The listing builds one solid part. Answer for the finished solid, in the listing's coordinates (mm). A direction names the side the tool comes from. Coordinates: 2 decimals unless noted, no trailing zeros. Write each loop counter-clockwise with the first axis right and the second up, starting at its lowest first coordinate (ties: lowest second). Pieces come first, ordered by that corner, then holes. Notation, with made-up numbers: M 70.5,35 L 111.5,35 A20 ccw 111.5,49 Z; hole C 16,-24 d11. An arc over 180 degrees is marked long. Put each result on its own line as item: value. Start each with the question number.
```python
from build123d import *

# Parameters (mm, degrees)
SKETCH1_W            = 25
SKETCH1_H            = 25
SKETCH1_W_2          = 9
SKETCH1_H_2          = 21
BOSS_EXTRUDE1_DEPTH  = 1.5
BOSS_EXTRUDE2_DEPTH  = 2
BOSS_EXTRUDE3_DEPTH  = 2
BOSS_EXTRUDE8_DEPTH  = 2
SKETCH12_W           = 2
SKETCH12_H           = 25
BOSS_EXTRUDE10_DEPTH = 5.93
SKETCH11_W           = 18
SKETCH11_H           = 25
SKETCH11_W_2         = 14
SKETCH11_H_2         = 21
BOSS_EXTRUDE11_DEPTH = 2
SKETCH13_W           = 9
SKETCH13_H           = 3.93
CUT_EXTRUDE2_DEPTH   = 24.5


with BuildPart() as part:
    # Sketch1 → Boss-Extrude1 (new body)
    with BuildSketch(Plane(origin=(0, 0, 0), x_dir=(1, 0, 0), z_dir=(0, 1, 0))):
        with Locations((0, -1)):
            Rectangle(SKETCH1_W, SKETCH1_H)
        with Locations((-6, -1)):
            Rectangle(SKETCH1_W_2, SKETCH1_H_2, mode=Mode.SUBTRACT)
        with Locations((6, -1)):
            Rectangle(SKETCH1_W_2, SKETCH1_H_2, mode=Mode.SUBTRACT)
    extrude(amount=BOSS_EXTRUDE1_DEPTH)

    # Sketch2 → Boss-Extrude2 (add)
    with BuildSketch(Plane(origin=(12.5, 0, 0), x_dir=(0, 0, -1), z_dir=(1, 0, 0))):
        Polygon((-9.5, 7.5), (-1, 7.5), (-1, 0), (1, 0), (1, 7.5), (7.5, 7.5), (7.5, 0), (11.5, 0), (11.5, 9.5), (-13.5, 9.5), (-13.5, 0), (-9.5, 0), align=None)
    extrude(amount=BOSS_EXTRUDE2_DEPTH)

    # Sketch3 → Boss-Extrude3 (add)
    with BuildSketch(Plane.ZY.offset(12.5)):
        Polygon((1, 0), (1, 7.2), (9.5, 7.2), (9.5, 0), (13.5, 0), (13.5, 9.5), (-11.5, 9.5), (-11.5, 0), (-7.5, 0), (-7.5, 7.2), (-1, 7.2), (-1, 0), align=None)
    extrude(amount=BOSS_EXTRUDE3_DEPTH)

    # Sketch10 → Boss-Extrude8 (add)
    with BuildSketch(Plane(origin=(0, 0, -11.5), x_dir=(-1, 0, 0), z_dir=(0, 0, -1))):
        Polygon((14.5, 9.5), (-14.5, 9.5), (-14.5, 6.5), (-0.948009726, 6.5), (-0.948009726, 0), (0.95, 0), (0.95, 6.5), (14.5, 6.5), align=None)
    extrude(amount=BOSS_EXTRUDE8_DEPTH)

    # Sketch12 → Boss-Extrude10 (add)
    with BuildSketch(Plane(origin=(0, 0, 0), x_dir=(-1, 0, 0), z_dir=(0, -1, 0))):
        with Locations((-8, -1)):
            Rectangle(SKETCH12_W, SKETCH12_H)
        with Locations((8, -1)):
            Rectangle(SKETCH12_W, SKETCH12_H)
    extrude(amount=BOSS_EXTRUDE10_DEPTH)

    # Sketch11 → Boss-Extrude11 (add)
    with BuildSketch(Plane(origin=(0, -5.93, 0), x_dir=(-1, 0, 0), z_dir=(0, -1, 0))):
        with Locations((0, -1)):
            Rectangle(SKETCH11_W, SKETCH11_H)
        with Locations((0, -1)):
            Rectangle(SKETCH11_W_2, SKETCH11_H_2, mode=Mode.SUBTRACT)
    extrude(amount=BOSS_EXTRUDE11_DEPTH)

    # Sketch13 → Cut-Extrude2 (cut, through all)
    with BuildSketch(Plane.ZY.offset(9)):
        with Locations((-5, -3.965)):
            Rectangle(SKETCH13_W, SKETCH13_H)
        with Locations((7, -3.965)):
            Rectangle(SKETCH13_W, SKETCH13_H)
    extrude(amount=-CUT_EXTRUDE2_DEPTH, mode=Mode.SUBTRACT)


solid = part.part
```
1) Determine the mould class of faces 1 (the face through (-8, -2, 7)), 2 (the face through (6, 1, -9.5)), 3 (the face through (-12, 0, 1)), 4 (the face through (0, 7, -11.5)) for opening direction Z: +Z half, -Z half, draft (parallel to the pull), parting line (faces both ways), or undercut.
2) For faces 5 (the face through (-7, -4, 1)), 6 (the face through (8, -5.93, -5)), 7 (the face through (-12.5, 1, -4)), determine the directions among +Z, -Z, +X, -X, +Y, -Y from which every point of the face is accessible in a straight line to the end or side of a thin tool.
3) A cutting plane is placed at C-C on x = 9.5. Write down the section's boundary in (y, z).
4) A cutting plane is placed at A-A on z = -8. State how many separate pieces and enclosed holes the cut face has, then the cut area to 3 significant figures.
5) Given pin 1 Ø1.6 at (x, y) = (-0.5, -6.5) entering from -Z; pin 2 Ø2 at (x, z) = (5.5, -3) entering from -Y; pin 3 Ø1.5 at (x, z) = (-2, -1) entering from +Y; pin 4 Ø8.5 at (y, z) = (-5.5, 4) entering from -X, each flat-ended and moving along its own axis, determine where each tip first touches the part or whether it passes through.
6) A cutting plane is placed at D-D on y = 3.25. Write down the section's boundary in (x, z), then the cut area to 3 significant figures.
7) A cutting plane is placed at B-B on y = -3.25. Write down the section's boundary in (x, z).
8) Straight lines are drawn through the part: probe 1 along X at (y, z) = (0.5, -5.5); probe 2 along Z at (x, y) = (-2, -6.75); probe 3 along X at (y, z) = (-1.75, -9.5). For each, find the intervals that lie inside material, in ascending order.
Answers follow:
1. face 1: undercut
1. face 2: undercut
1. face 3: draft
1. face 4: +Z half
2. face 5: none
2. face 6: +X, -X
2. face 7: -X, -Y
3. outline: M 0,-11.5 L 1.5,-11.5 L 1.5,-9.5 L 0,-9.5 Z; M 0,11.5 L 1.5,11.5 L 1.5,13.5 L 0,13.5 Z; M 6.5,-13.5 L 9.5,-13.5 L 9.5,-11.5 L 6.5,-11.5 Z
4. separate pieces: 7
4. enclosed holes: 0
4. area: 64.5 mm²
5. pin 1: stops at z = -11.5
5. pin 2: passes through
5. pin 3: stops at y = 1.5
5. pin 4: stops at x = -9
6. outline: M -14.5,-11.5 L -12.5,-11.5 L -12.5,-7.5 L -14.5,-7.5 Z; M -14.5,-1 L -12.5,-1 L -12.5,1 L -14.5,1 Z; M -14.5,9.5 L -12.5,9.5 L -12.5,13.5 L -14.5,13.5 Z; M -0.95,-13.5 L 0.95,-13.5 L 0.95,-11.5 L -0.95,-11.5 Z; M 12.5,-11.5 L 14.5,-11.5 L 14.5,-7.5 L 12.5,-7.5 Z; M 12.5,-1 L 14.5,-1 L 14.5,1 L 12.5,1 Z; M 12.5,9.5 L 14.5,9.5 L 14.5,13.5 L 12.5,13.5 Z
6. area: 43.8 mm²
7. outline: M -9,-11.5 L -7,-11.5 L -7,-9.5 L -9,-9.5 Z; M -9,-0.5 L -7,-0.5 L -7,2.5 L -9,2.5 Z; M -9,11.5 L -7,11.5 L -7,13.5 L -9,13.5 Z; M 7,-11.5 L 9,-11.5 L 9,-9.5 L 7,-9.5 Z; M 7,-0.5 L 9,-0.5 L 9,2.5 L 7,2.5 Z; M 7,11.5 L 9,11.5 L 9,13.5 L 7,13.5 Z
8. probe 1: x = -12.5 to -10.5, -1.5 to 1.5, 10.5 to 12.5
8. probe 2: z = -11.5 to -9.5, 11.5 to 13.5
8. probe 3: x = -9 to -7, 7 to 9
